Could you check a few things on this model? Use its own coordinates, in mm. A direction names the side the tool comes from. Round coordinates to 2 decimals unless told otherwise and drop trailing zeros. Loops run counter-clockwise (first coordinate to the right, second up) from the corner with the lowest first, then second, coordinate; pieces in that order, holes last. Notation, with made-up numbers: (52, 55) - (102, 55) arc R8 ccw to (102, 69) - close; hole circle Ø7 at (48.5, -34.5). An arc over 180 degrees is marked (long way). Answer as CSV lines item,"result". Start each with the question number.
1) Please list where these lines run through material, in increasing order: line 1 along Y through (x, z) = (78.5, 7.5); line 2 along Y through (x, z) = (14, 7.5); line 3 along X through (y, z) = (-40.5, 4.75).
2) Suppose I cut it at A-A, the plane y = -8.5. Write out the boundary of the cut face in (x, z), then the cut area to 3 significant figures.
3) I'm going to push flat-ended pins straight in: pin 1 Ø4.5 at (x, y) = (78.5, -58) entering from +Z; pin 2 Ø0.8 at (x, z) = (-21, 2.5) entering from +Y; pin 3 Ø3.5 at (x, y) = (-78.5, 56.5) entering from +Z. Where does each tip first touch, or does it pass through?
4) Suppose I cut it at C-C, the plane x = -60.5. Write out the boundary of the cut face in (y, z), then the cut area to 3 significant figures.
5) Suppose I cut it at D-D, the plane y = 44. Write out the boundary of the cut face in (x, z), then the cut area to 3 significant figures.
6) We'd pull the mould along Z, two halves only. Please class faces 4 (the face through (-78, -58, 2)), 5 (the face through (-23, 62.8, 10.7)), 6 (the face through (-22.09, 66.02, 9.22)), 7 (the face through (-2, 61.5, 15)): pulls with the +Z half, pulls with the -Z half, needs draft (parallel to the pull), parting line crosses it, or undercut.
7) Which directions (+Z, -Z, +X, -X, +Y, -Y) give clear straight access to the entire face, cutting with the end or side of a thin tool? Please do faces 1 (the face through (-14.5, 42.4, 0)), 2 (the face through (53, 48, 7)), 3 (the face through (21.7, 64.5, 10.5)).
8) Suppose I cut it at B-B, the plane x = 20. Count the separate pieces of the cut face and the enclosed holes in it, then the cut area to 3 significant figures.
```python
from build123d import *

# Parameters (mm, degrees)
CROQUIS1_W              = 218
CROQUIS1_H              = 145
SALIENTE_EXTRUIR1_DEPTH = 10
CORTAR_EXTRUIR1_DEPTH   = 7
CROQUIS3_W              = 157.5
CROQUIS3_H              = 90
CORTAR_EXTRUIR2_DEPTH   = 132.096338622
CHAFL_N1_SIZE           = 2
CORTAR_EXTRUIR3_START   = -2
CROQUIS4_R              = 1.95
CORTAR_EXTRUIR3_DEPTH   = 130.290707973
CROQUIS5_W              = 50
CROQUIS5_H              = 12
CORTAR_EXTRUIR4_DEPTH   = 7
CHAFL_N3_SIZE           = 1
CROQUIS6_OUTSIDE_W      = 272.402
CROQUIS6_OUTSIDE_H      = 199.402
CROQUIS6_OUTSIDE_W_2    = 175.5
CROQUIS6_OUTSIDE_H_2    = 130.5
CORTAR_EXTRUIR5_DEPTH   = 132.290707973
CROQUIS7_W              = 175.5
CROQUIS7_H              = 130.5
CROQUIS7_W_2            = 169.5
CROQUIS7_H_2            = 124.5
SALIENTE_EXTRUIR2_DEPTH = 10
CHAFL_N4_SIZE           = 2
CHAFL_N5_SIZE           = 1
CORTAR_EXTRUIR6_REACH   = 190.564
CROQUIS8_W              = 11
CROQUIS8_H              = 50
CROQUIS9_W              = 60
CROQUIS9_H              = 16
SALIENTE_EXTRUIR3_DEPTH = 3
CHAFL_N6_SIZE           = 3
CORTAR_EXTRUIR7_REACH   = 163.689
CROQUIS10_R             = 2.1
CORTAR_EXTRUIR8_REACH   = 166.689
CORTAR_EXTRUIR8_START   = -3


with BuildPart() as part:
    # Croquis1 → Saliente-Extruir1 (new body)
    with BuildSketch(Plane.XY):
        Rectangle(CROQUIS1_W, CROQUIS1_H)
    extrude(amount=SALIENTE_EXTRUIR1_DEPTH)

    # Croquis2 → Cortar-Extruir1 (cut)
    with BuildSketch(Plane.XY.offset(10)):
        Polygon((-83, 43), (-83, 48), (82.7, 48), (82.7, -53), (80.5, -53), (-83, -53), align=None)
    extrude(amount=-CORTAR_EXTRUIR1_DEPTH, mode=Mode.SUBTRACT)

    # Croquis3 → Cortar-Extruir2 (cut, through all)
    with BuildSketch(Plane.XY.offset(3)):
        with Locations((-1.25, -5)):
            Rectangle(CROQUIS3_W, CROQUIS3_H)
    extrude(amount=-CORTAR_EXTRUIR2_DEPTH, mode=Mode.SUBTRACT)

    # Chaflán1
    chafl_n1_edges = [part.edges().sort_by_distance(p)[0] for p in [
        (-80, -5, 0),
        (-1.25, 40, 0),
        (77.5, -5, 0),
        (-1.25, -50, 0),
    ]]
    chamfer(chafl_n1_edges, length=CHAFL_N1_SIZE)

    # Croquis4 → Cortar-Extruir3 (cut, through all)
    with BuildSketch(Plane(origin=(0, 0, 0), x_dir=(-1, 0, 0), z_dir=(0, 0, -1)).offset(CORTAR_EXTRUIR3_START)):
        with Locations((-78.5, 56.5)):
            Circle(CROQUIS4_R)
        with Locations((78.5, 56.5)):
            Circle(CROQUIS4_R)
        with Locations((78.5, -58)):
            Circle(CROQUIS4_R)
        with Locations((-78.5, -58)):
            Circle(CROQUIS4_R)
    extrude(amount=-CORTAR_EXTRUIR3_DEPTH, mode=Mode.SUBTRACT)

    # Croquis5 → Cortar-Extruir4 (cut)
    with BuildSketch(Plane.XY.offset(10)):
        with Locations((0, 54)):
            Rectangle(CROQUIS5_W, CROQUIS5_H)
        with Locations((0, -54)):
            Rectangle(CROQUIS5_W, CROQUIS5_H)
    extrude(amount=-CORTAR_EXTRUIR4_DEPTH, mode=Mode.SUBTRACT)

    # Chaflán3
    chafl_n3_edges = [part.edges().sort_by_distance(p)[0] for p in [
        (80.45, -58, 10),
        (-76.55, -58, 10),
        (-76.55, 56.5, 10),
        (80.45, 56.5, 10),
    ]]
    chamfer(chafl_n3_edges, length=CHAFL_N3_SIZE)

    # Croquis6 outside → Cortar-Extruir5 (cut, through all)
    with BuildSketch(Plane.XY.offset(10)):
        Rectangle(CROQUIS6_OUTSIDE_W, CROQUIS6_OUTSIDE_H)
        with Locations((-1.25, -0.75)):
            Rectangle(CROQUIS6_OUTSIDE_W_2, CROQUIS6_OUTSIDE_H_2, mode=Mode.SUBTRACT)
    extrude(amount=-CORTAR_EXTRUIR5_DEPTH, mode=Mode.SUBTRACT)

    # Croquis7 → Saliente-Extruir2 (add)
    with BuildSketch(Plane.XY.offset(10)):
        with Locations((-1.25, -0.75)):
            Rectangle(CROQUIS7_W, CROQUIS7_H)
        with Locations((-1.25, -0.75)):
            Rectangle(CROQUIS7_W_2, CROQUIS7_H_2, mode=Mode.SUBTRACT)
    extrude(amount=SALIENTE_EXTRUIR2_DEPTH)

    # Chaflán4
    chafl_n4_edges = [part.edges().sort_by_distance(p)[0] for p in [
        (-89, 64.5, 10),
        (86.5, 64.5, 10),
        (86.5, -66, 10),
        (-89, -66, 10),
    ]]
    chamfer(chafl_n4_edges, length=CHAFL_N4_SIZE)

    # Chaflán5
    chafl_n5_edges = [part.edges().sort_by_distance(p)[0] for p in [
        (86.5, -0.75, 0),
        (-1.25, 64.5, 0),
        (-89, -0.75, 0),
        (-1.25, -66, 0),
        (-88, 63.5, 0),
        (-88, -65, 0),
        (85.5, -65, 0),
        (85.5, 63.5, 0),
    ]]
    chamfer(chafl_n5_edges, length=CHAFL_N5_SIZE)

    # Croquis8 → Cortar-Extruir6 (cut, up to next)
    with BuildSketch(Plane(origin=(86.5, 0, 0), x_dir=(0, 0, -1), z_dir=(1, 0, 0)), mode=Mode.PRIVATE) as cortar_extruir6_sk1:
        with Locations((-14.5, -28)):
            Rectangle(CROQUIS8_W, CROQUIS8_H)
    cortar_extruir6_tool1 = extrude(cortar_extruir6_sk1.sketch, amount=-CORTAR_EXTRUIR6_REACH, mode=Mode.PRIVATE) & part.part
    add(cortar_extruir6_tool1.solids().sort_by_distance((86.5, -28, 14.5))[0], mode=Mode.SUBTRACT)

    # Croquis9 → Saliente-Extruir3 (add)
    with BuildSketch(Plane(origin=(0, 64.5, 0), x_dir=(1, 0, 0), z_dir=(0, 1, 0))):
        with Locations((0, -9)):
            Rectangle(CROQUIS9_W, CROQUIS9_H)
    extrude(amount=SALIENTE_EXTRUIR3_DEPTH)

    # Chaflán6
    chafl_n6_edges = [part.edges().sort_by_distance(p)[0] for p in [
        (0, 67.5, 17),
        (-30, 67.5, 9),
        (0, 67.5, 1),
        (30, 67.5, 9),
    ]]
    chamfer(chafl_n6_edges, length=CHAFL_N6_SIZE - 0.0001)  # a hair under: the kernel refuses the full size

    # Croquis10 → Cortar-Extruir7 (cut, up to next)
    with BuildSketch(Plane(origin=(0, 67.5, 0), x_dir=(1, 0, 0), z_dir=(0, 1, 0)), mode=Mode.PRIVATE) as cortar_extruir7_sk1:
        with Locations(Location((20, -9, 0), (0, 0, 270))):
            Circle(CROQUIS10_R)
    cortar_extruir7_tool1 = extrude(cortar_extruir7_sk1.sketch, amount=-CORTAR_EXTRUIR7_REACH, mode=Mode.PRIVATE) & part.part
    # Croquis10 → Cortar-Extruir7 (cut, up to next)
    with BuildSketch(Plane(origin=(0, 67.5, 0), x_dir=(1, 0, 0), z_dir=(0, 1, 0)), mode=Mode.PRIVATE) as cortar_extruir7_sk2:
        with Locations(Location((-20, -9, 0), (0, 0, 208.436890149))):
            Circle(CROQUIS10_R)
    cortar_extruir7_tool2 = extrude(cortar_extruir7_sk2.sketch, amount=-CORTAR_EXTRUIR7_REACH, mode=Mode.PRIVATE) & part.part
    add(cortar_extruir7_tool1.solids().sort_by_distance((20, 67.5, 9))[0], mode=Mode.SUBTRACT)
    add(cortar_extruir7_tool2.solids().sort_by_distance((-20, 67.5, 9))[0], mode=Mode.SUBTRACT)

    # Croquis11 → Cortar-Extruir8 (cut, up to next)
    with BuildSketch(Plane(origin=(0, 67.5, 0), x_dir=(1, 0, 0), z_dir=(0, 1, 0)).offset(CORTAR_EXTRUIR8_START), mode=Mode.PRIVATE) as cortar_extruir8_sk1:
        Polygon((23.983716857, -9), (21.991858429, -5.55), (18.008141571, -5.55), (16.016283143, -9), (18.008141571, -12.45), (21.991858429, -12.45), align=None)
    cortar_extruir8_tool1 = extrude(cortar_extruir8_sk1.sketch, amount=-CORTAR_EXTRUIR8_REACH, mode=Mode.PRIVATE) & part.part
    # Croquis11 → Cortar-Extruir8 (cut, up to next)
    with BuildSketch(Plane(origin=(0, 67.5, 0), x_dir=(1, 0, 0), z_dir=(0, 1, 0)).offset(CORTAR_EXTRUIR8_START), mode=Mode.PRIVATE) as cortar_extruir8_sk2:
        Polygon((-16.016283143, -9), (-18.008141571, -5.55), (-21.991858429, -5.55), (-23.983716857, -9), (-21.991858429, -12.45), (-18.008141571, -12.45), align=None)
    cortar_extruir8_tool2 = extrude(cortar_extruir8_sk2.sketch, amount=-CORTAR_EXTRUIR8_REACH, mode=Mode.PRIVATE) & part.part
    add(cortar_extruir8_tool1.solids().sort_by_distance((20, 64.5, 9))[0], mode=Mode.SUBTRACT)
    add(cortar_extruir8_tool2.solids().sort_by_distance((-20, 64.5, 9))[0], mode=Mode.SUBTRACT)


solid = part.part
```
Filled sheet:
1,line 1,"-66 to -59.95, -56.05 to -53, 48 to 54.55, 58.45 to 64.5"
1,line 2,"-66 to -60, 60 to 67.5"
1,line 3,"-89 to -83, 82.7 to 86.5"
2,outline,"(-89, 1) - (-88, 0) - (-82, 0) - (-80, 2) - (-80, 3) - (-83, 3) - (-83, 10) - (-86, 10) - (-86, 20) - (-89, 20) - close; (77.5, 2) - (79.5, 0) - (85.5, 0) - (86.5, 1) - (86.5, 9) - (82.7, 9) - (82.7, 3) - (77.5, 3) - close"
2,area,"144 mm²"
3,pin 1,"z = 9.3"
3,pin 2,"y = 66.4"
3,pin 3,"z = 2"
4,outline,"(-66, 1) - (-65, 0) - (-52, 0) - (-50, 2) - (-50, 3) - (-53, 3) - (-53, 10) - (-63, 10) - (-63, 20) - (-66, 20) - close; (40, 2) - (42, 0) - (63.5, 0) - (64.5, 1) - (64.5, 20) - (61.5, 20) - (61.5, 10) - (48, 10) - (48, 3) - (40, 3) - close"
4,area,"383 mm²"
5,outline,"(-89, 1) - (-88, 0) - (85.5, 0) - (86.5, 1) - (86.5, 20) - (83.5, 20) - (83.5, 10) - (82.7, 10) - (82.7, 3) - (-83, 3) - (-83, 10) - (-86, 10) - (-86, 20) - (-89, 20) - close"
5,area,"654 mm²"
6,face 4,"pulls with the +Z half"
6,face 5,"undercut"
6,face 6,"undercut"
6,face 7,"needs draft"
7,face 1,"-Z, +X, -X, +Y, -Y"
7,face 2,"+Z"
7,face 3,"none"
8,separate pieces,"3"
8,enclosed holes,"0"
8,area,"249 mm²"
